Part model, mm, in its own coordinate system. Face numbers are marked on the shaded views. A direction names the side the tool comes from. Coordinates: 2 decimals unless noted, no trailing zeros. Order: outer loops, then holes, each group sorted by start corner. A loop starts at its lowest first (then second) coordinate and runs counter-clockwise, first axis right, second up.
Autodesk Inventor part; units mm, degrees
ref_plane "YZ Plane" through (0, 0, 0) normal (1, 0, 0) x (0, 1, 0)
ref_plane "XZ Plane" through (0, 0, 0) normal (0, 1, 0) x (-1, 0, 0)
ref_plane "XY Plane" through (0, 0, 0) normal (0, 0, 1) x (1, 0, 0)
sketch "Sketch1" plane through (0, 0, 0) normal (0, 0, 1) x (1, 0, 0)
  line L0 (0, 0) -> (36.8826, 0)
  line L1 (36.8826, 0) -> (36.8826, 40)
  line L2 (0, 40) -> (36.8826, 40)
  line L3 (0, 0) -> (0, 40)
  line L4 (-21.6348, 40) -> (-58.5174, 40)
  line L5 (-58.5174, 40) -> (-58.5174, 0)
  line L6 (-21.6348, 0) -> (-58.5174, 0)
  line L7 (-21.6348, 40) -> (-21.6348, 0)
  line L8 (-21.6348, -8) -> (-58.5174, -8)
  line L9 (-58.5174, -8) -> (-58.5174, -48)
  line L10 (-21.6348, -48) -> (-58.5174, -48)
  line L11 (-21.6348, -8) -> (-21.6348, -48)
  line L12 (0, -48) -> (36.8826, -48)
  line L13 (36.8826, -48) -> (36.8826, -8)
  line L14 (0, -8) -> (36.8826, -8)
  line L15 (0, -48) -> (0, -8)
  line L16 (21.8826, 32) -> (-43.5174, 32)
  line L17 (-43.5174, 32) -> (-43.5174, -40)
  line L18 (-43.5174, -40) -> (21.8826, -40)
  line L19 (21.8826, -40) -> (21.8826, 32)
  dimension "d0" = 8
  dimension "d1" = 8
  dimension "d2" = 15
  dimension "d3" = 15
extrude "Extrusion1" add sketch "Sketch1" along normal blind 5 contours L3 L16 L19 L0 | L0 L19 L14 L15 L18 L11 L8 L17 L6 L7 L16 L3 | L19 L18 L15 L14 | L7 L6 L17 L16 | L18 L17 L8 L11
sketch "Sketch2" plane through (0, 0, 0) normal (0, 0, -1) x (-1, 0, 0)
  line L0 (0, -48) -> (-36.8826, -48)
  line L1 (-36.8826, -48) -> (-36.8826, -8)
  line L2 (0, -8) -> (-36.8826, -8)
  line L3 (0, -48) -> (0, -8)
  line L4 (0, 0) -> (-36.8826, 0)
  line L5 (-36.8826, 0) -> (-36.8826, 40)
  line L6 (0, 40) -> (-36.8826, 40)
  line L7 (0, 0) -> (0, 40)
  line L8 (21.6348, 40) -> (58.5174, 40)
  line L9 (58.5174, 40) -> (58.5174, 0)
  line L10 (21.6348, 0) -> (58.5174, 0)
  line L11 (21.6348, 40) -> (21.6348, 0)
  line L12 (21.6348, -8) -> (58.5174, -8)
  line L13 (58.5174, -8) -> (58.5174, -48)
  line L14 (21.6348, -48) -> (58.5174, -48)
  line L15 (21.6348, -8) -> (21.6348, -48)
  line L16 (0, -38) -> (21.6348, -38)
  line L17 (21.6348, -38) -> (21.6348, -18)
  line L18 (21.6348, -18) -> (0, -18)
  line L19 (0, -18) -> (0, -38)
  line L20 (0, 10) -> (21.6348, 10)
  line L21 (21.6348, 10) -> (21.6348, 30)
  line L22 (21.6348, 30) -> (0, 30)
  line L23 (0, 30) -> (0, 10)
  point P0 (0, 30)
  point P1 (0, -18)
  dimension "d6" = 20
  dimension "d7" = 20
  dimension "d8" = 10
  dimension "d9" = 10
extrude "Extrusion2" add sketch "Sketch2" along normal blind 20 contours L3 L18 L15 L16 | L7 L22 L11 L20
sketch "Sketch3" plane through (0, 0, 5) normal (0, 0, 1) x (1, 0, 0)
  circle A0 centre (10.1826, 17) radius 2.5
  circle A1 centre (-31.8174, 17) radius 2.5
  circle A2 centre (10.1826, -25) radius 2.5
  circle A3 centre (-31.8174, -25) radius 2.5
  line L0 (21.8826, -40) -> (21.8826, 32)
  line L1 (-43.5174, 32) -> (-43.5174, -40)
  line L2 (10.1826, 17) -> (-31.8174, 17)
  line L3 (10.1826, -25) -> (-31.8174, -25)
  line L4 (21.8826, 32) -> (-43.5174, 32)
  line L5 (-43.5174, -40) -> (21.8826, -40)
  point P0 (0, 0)
  point P1 (-10.8174, 17)
  point P2 (-10.8174, 32)
  point P3 (-10.8174, -25)
  point P4 (-10.8174, -40)
  dimension "d12" = 5
  dimension "d13" = 5
  dimension "d14" = 5
  dimension "d15" = 5
  dimension "d16" = 42
  dimension "d17" = 42
  dimension "d18" = 15
  dimension "d19" = 15
extrude "Extrusion3" cut sketch "Sketch3" against normal through all contours A0 | A1 | A2 | A3
sketch "Sketch4" plane through (0, -38, 0) normal (1, 0, 0) x (0, 0, -1)
  arc A0 (2.5, 58) -> (5, 53.6699) centre (7.5, 58) ccw
  arc A1 (5, 53.6699) -> (10, 53.6699) centre (7.5, 58) ccw
  arc A2 (10, 53.6699) -> (12.5, 58) centre (7.5, 58) ccw
  arc A3 (12.5, 58) -> (10, 62.3301) centre (7.5, 58) ccw
  arc A4 (10, 62.3301) -> (5, 62.3301) centre (7.5, 58) ccw
  arc A5 (5, 62.3301) -> (2.5, 58) centre (7.5, 58) ccw
  circle A6 centre (7.5, 58) radius 3.1
  arc A7 (2.3201, 9.9991) -> (4.8201, 5.669) centre (7.3201, 9.9991) ccw
  arc A8 (4.8201, 5.669) -> (9.8201, 5.669) centre (7.3201, 9.9991) ccw
  arc A9 (9.8201, 5.669) -> (12.3201, 9.9991) centre (7.3201, 9.9991) ccw
  arc A10 (12.3201, 9.9991) -> (9.8201, 14.3292) centre (7.3201, 9.9991) ccw
  arc A11 (9.8201, 14.3292) -> (4.8201, 14.3292) centre (7.3201, 9.9991) ccw
  arc A12 (4.8201, 14.3292) -> (2.3201, 9.9991) centre (7.3201, 9.9991) ccw
  circle A13 centre (7.3201, 9.9991) radius 3.1
  circle A14 centre (13.5, 58) radius 3.5
  circle A15 centre (13.5, 9.9991) radius 3.5
  line L0 (0, -2) -> (0, 70)
  point P0 (0, 38)
  dimension "d24" = 7
  dimension "d25" = 7
  dimension "d26" = 10
  dimension "d27" = 10
extrude "Extrusion5" cut sketch "Sketch4" against normal through all contours A14 A6 A3 A2 | A2 A3 A14 | A14 A6 | A15 A13 A10 A9 | A9 A10 A15 | A15 A13 picked at (10.2115, 57.6094) picked at (10.1547, 9.9991)
properties part number "bearing support"
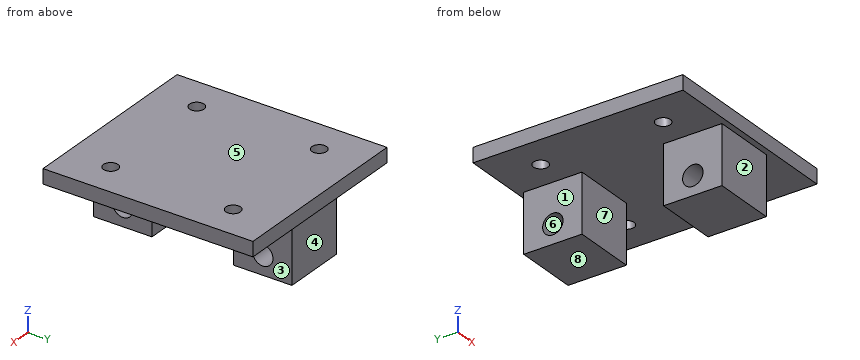
(1) Drop flat-ended pins along their axis: pin 1 (6 mm diameter, centred on y = 24.5, z = -9, fed in from -X); pin 2 (4.5 mm diameter, centred on x = -31.82, y = 17, fed in from -Z); pin 3 (6 mm diameter, centred on x = -34.5, z = -2, fed in from -Y); pin 4 (8 mm diameter, centred on x = -36.5, y = -28.5, fed in from -Z). Give the stop position or say it passes through.
(2) Slice it at A-A, the plane z = -4. Give the cut face in (x, y), then the cut area to 3 significant figures.
(3) Slice it at D-D, the plane x = -14. Give the cut face in (y, z), then the cut area to 3 significant figures.
(4) Probe line 1 (Y direction, x = -9, z = -13.5); line 2 (Y direction, x = -18, z = -15.75); line 3 (Y direction, x = -8, z = -0.25). List the from-to ranges inside material, lowest first.
(5) Tool access for the marked faces 1, 2, 3 and 4: list every direction of +Z, -Z, +X, -X, +Y, -Y with a clear straight run to the whole face (end or side of a thin tool).
(6) Slice it at B-B, the plane z = -13.5. Give the cut face in (x, y), then the cut area to 3 significant figures.
(7) Slice it at C-C, the plane x = -31. Give the cut face in (y, z).
(8) Pull direction Z, two halves, no side cores. Call the marked faces 5, 6, 7 and 8: +Z half, -Z half, draft (parallel to the pull), parting line (faces both ways), or undercut.
Here are the results:
1. pin 1: stops at x = -21.63
1. pin 2: passes through
1. pin 3: stops at y = -40
1. pin 4: stops at z = 0
2. outline: (-21.63, -38) - (0, -38) - (0, -18) - (-21.63, -18) - close; (-21.63, 10) - (0, 10) - (0, 30) - (-21.63, 30) - close
2. area: 865 mm2
3. outline: (-40, 0) - (-38, 0) - (-38, -20) - (-18, -20) - (-18, 0) - (10, 0) - (10, -20) - (30, -20) - (30, 0) - (32, 0) - (32, 5) - (-40, 5) - close; hole circle Ø7 at (-28, -13.5); hole circle Ø7 at (20, -13.5)
3. area: 1,080 mm2
4. line 1: y = -38 to -31.5, -24.5 to -18, 10 to 16.5, 23.5 to 30
4. line 2: y = -38 to -30.68, -25.32 to -18, 10 to 17.32, 22.68 to 30
4. line 3: y = -38 to -18, 10 to 30
5. face 1: -Z, -X, +Y, -Y
5. face 2: -Z, +X, -X, -Y
5. face 3: -Z, +X, +Y, -Y
5. face 4: -Z, +X, -X, +Y
6. outline: (-21.63, -38) - (0, -38) - (0, -31.5) - (-21.63, -31.5) - close; (-21.63, -24.5) - (0, -24.5) - (0, -18) - (-21.63, -18) - close; (-21.63, 10) - (0, 10) - (0, 16.5) - (-21.63, 16.5) - close; (-21.63, 23.5) - (0, 23.5) - (0, 30) - (-21.63, 30) - close
6. area: 563 mm2
7. outline: (-40, 0) - (-27.36, 0) - (-27.36, 5) - (-40, 5) - close; (-22.64, 0) - (14.64, 0) - (14.64, 5) - (-22.64, 5) - close; (19.36, 0) - (32, 0) - (32, 5) - (19.36, 5) - close
8. face 5: +Z half
8. face 6: undercut
8. face 7: draft
8. face 8: -Z half
